Here's how the part is built. I have some questions about the finished solid (model axes, mm). Coordinates: 2 decimals unless noted, no trailing zeros. Write each loop counter-clockwise with the first axis right and the second up, starting at its lowest first coordinate (ties: lowest second). Pieces come first, ordered by that corner, then holes. Notation, with made-up numbers: M 25.5,63 L 71.5,63 A32 cw 71.5,89 Z; hole C 10,-15 d1. An arc over 180 degrees is marked long. Use a Markdown table: item, result.
Autodesk Inventor part; units mm, degrees
ref_plane "Work Plane1" through (-42.7075, 0, 0) normal (1, 0, 0) x (0, 0, -1)
ref_plane "Work Plane2" through (-42.7075, 0, -90) normal (-1, 0, 0) x (0, 0, 1)
ref_plane "YZ Plane" through (0, 0, 0) normal (1, 0, 0) x (0, 1, 0)
sketch "Sketch1" plane through (0, 0, 0) normal (0, 1, 0) x (-1, 0, 0)
  line L0 (0, 0) -> (85.415, 0)
  line L1 (85.415, 0) -> (85.415, -90)
  line L2 (85.415, -90) -> (0, -90)
  line L3 (0, -90) -> (0, 0)
  dimension "d0" = 85.415
  dimension "d1" = 90
extrude "Extrusion1" add sketch "Sketch1" along normal blind 4
ref_plane "Work Plane1" through (-42.7075, 0, 0) normal (1, 0, 0) x (0, 0, -1)
ref_plane "Work Plane2" through (-42.7075, 0, -90) normal (-1, 0, 0) x (0, 0, 1)
sketch "Sketch5" plane through (-42.7075, 0, -90) normal (-1, 0, 0) x (0, 0, 1)
  line L0 (90, 0) -> (90, 4) construction
  line L1 (90, 4) -> (96.1, 4) construction
  line L2 (96.1, 4) -> (96.1, 21.2) construction
  line L3 (96.1, 21.2) -> (90, 21.2) construction
  line L4 (90, 21.2) -> (90, 4) construction
  circle A0 centre (96.1, 21.2) radius 4.5
  line L5 (90, 0) -> (0, 0)
  line L6 (0, 0) -> (0, 4)
  line L7 (90, 4) -> (0, 4)
  line L8 (90, 0) -> (90, 4)
  line L9 (91.6189, 21.6119) -> (90.4175, 8.5423)
  line L10 (99.0878, 4.5423) -> (100.5811, 20.7881)
  line L11 (90, 0) -> (90, 4)
  line L12 (90, 0) -> (94.1088, 0)
  line L13 (85.4385, 4) -> (75.881, 4)
  line L14 (90, 4) -> (0, 4)
  arc A1 (85.4385, 4) -> (90.4175, 8.5423) centre (85.4385, 9) ccw
  arc A2 (94.1088, 0) -> (99.0878, 4.5423) centre (94.1088, 5) ccw
  point P0 (92.3607, 23.7035)
  dimension "d14" = 6.1
  dimension "d15" = 17.2
  dimension "d16" = 9
  dimension "d29" = 5
extrude "Extrusion4" add sketch "Sketch5" along normal blind 10 contours A0 | A0 L10 A2 L12 L8 L7 A1 L9
sketch "Sketch6" plane through (-42.7075, 0, -90) normal (1, 0, 0) x (0, 0, -1)
  arc A0 (-91.6189, 21.6119) -> (-100.5811, 20.7881) centre (-96.1, 21.2) ccw
  circle A1 centre (-96.1, 21.2) radius 2.3
  point P0 (-90, 0)
  point P1 (-99.8393, 18.6965)
  point P2 (-92.3607, 23.7035)
  dimension "d19" = 4.6
extrude "Extrusion5" cut sketch "Sketch6" against normal blind 3.1
sketch "Sketch7" plane through (-52.7075, 0, -90) normal (-1, 0, 0) x (0, 0, 1)
  arc A0 (100.5811, 20.7881) -> (91.6189, 21.6119) centre (96.1, 21.2) ccw
  circle A1 centre (96.1, 21.2) radius 2.3
  point P0 (90, 0)
  point P1 (99.8393, 18.6965)
  point P2 (92.3607, 23.7035)
  dimension "d22" = 4.6
extrude "Extrusion6" cut sketch "Sketch7" against normal blind 3.1
sketch "Sketch8" plane through (-49.6075, 21.2, 6.1) normal (-1, 0, 0) x (0, 0, 1)
  circle A0 centre (0, 0) radius 2.3
  circle A1 centre (0, 0) radius 1
  point P0 (-6.1, -21.2)
  dimension "d25" = 2
extrude "Extrusion7" cut sketch "Sketch8" against normal through all contours A1
fillet "Fillet2" radius 5 4 edges at (-85.415, 2, 0) (0, 2, 0) (0, 2, -90) (-85.415, 2, -90)
properties part number "Tapas" material "ABS Plastic"
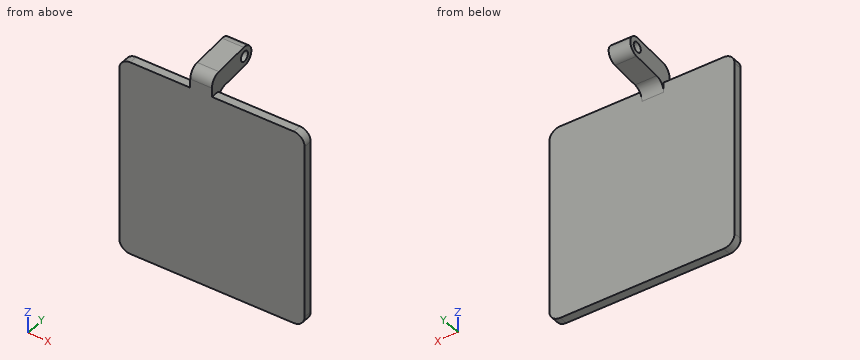
1. I need wall thicknesses on probe 1 along Y at (x, z) = (-50.4, 6.1); probe 2 along Y at (x, z) = (-47.65, 6.1); probe 3 along Y at (x, z) = (-39, -64). Which ranges of each line are inside material? Lowest first, please.
Answers follow:
| item | result |
|---|---|
| probe 1 | y = 0.41 to 18.9, 23.5 to 25.7 |
| probe 2 | y = 0.41 to 20.2, 22.2 to 25.7 |
| probe 3 | y = 0 to 4 |
2. Suppose I cut it at C-C on y = 16.5. Write out the boundary of the cut face in (x, z), and give its area (3 significant figures).
Answers follow:
| item | result |
|---|---|
| outline | M -52.71,1.15 L -42.71,1.15 L -42.71,10.19 L -52.71,10.19 Z |
| area | 90.4 mm2 |
3. Suppose I cut it at A-A on y = 2.75. Write out the boundary of the cut face in (x, z) (1 decimal).
Answers follow:
| item | result |
|---|---|
| outline | M -85.4,-85 A5 ccw -80.4,-90 L -5,-90 A5 ccw 0,-85 L 0,-5 A5 ccw -5,0 L -42.7,0 L -42.7,8.6 L -52.7,8.6 L -52.7,0 L -80.4,0 A5 ccw -85.4,-5 Z |
4. Suppose I cut it at B-B on x = -12.5. Write out the boundary of the cut face in (y, z).
Answers follow:
| item | result |
|---|---|
| outline | M 0,-90 L 4,-90 L 4,0 L 0,0 Z |
5. Will these pins go through, and if not, where does the flat tip stop? pin 1 Ø7.5 at (y, z) = (21.2, 6.1) entering from -X; pin 2 Ø2 at (x, z) = (-24, -23) entering from +Y; pin 3 Ø3 at (x, y) = (-61, 1.5) entering from +Z.
Answers follow:
| item | result |
|---|---|
| pin 1 | stops at x = -52.71 |
| pin 2 | stops at y = 4 |
| pin 3 | stops at z = 0 |
